Part model, mm, in its own coordinate system. A direction names the side the tool comes from. Give positions to 0.01 mm unless a question says otherwise; leave off trailing zeros. Order: outer loops, then holes, each group sorted by start corner. A loop starts at its lowest first (then second) coordinate and runs counter-clockwise, first axis right, second up. Notation, with made-up numbers: M 65,13 L 97,13 A12 cw 97,33 Z; hole C 1,-11.5 d6. An arc over 180 degrees is marked long. Return JSON: item names as keys, results as strings.
Autodesk Inventor part; units mm, degrees
ref_plane "YZ Plane" through (0, 0, 0) normal (1, 0, 0) x (0, 1, 0)
ref_plane "XZ Plane" through (0, 0, 0) normal (0, 1, 0) x (-1, 0, 0)
ref_plane "XY Plane" through (0, 0, 0) normal (0, 0, 1) x (1, 0, 0)
sketch "Sketch1" plane through (0, 0, 0) normal (0, 1, 0) x (-1, 0, 0)
  line L0 (0, 0) -> (68, 0)
  line L1 (68, 0) -> (68, -93)
  line L2 (68, -93) -> (0, -93)
  line L3 (0, -93) -> (0, 0)
  dimension "d0" = 93
  dimension "d1" = 68
extrude "Extrusion1" add sketch "Sketch1" along normal blind 8
fillet "Fillet1" radius 5 2 edges at (0, 4, -93) (-68, 4, -93)
fillet "Fillet2" radius 5 2 edges at (-68, 4, 0) (0, 4, 0)
sketch "Sketch2" plane through (0, 0, 0) normal (0, -1, 0) x (1, 0, 0)
  circle A0 centre (-7.8137, -81.5) radius 4
  circle A1 centre (-60.1863, -81.5) radius 4
  circle A2 centre (-60.1863, -11.5) radius 4
  circle A3 centre (-7.8137, -11.5) radius 4
  circle A4 centre (-34, -36) radius 4
  point P0 (0, 0)
  dimension "d27" = 70
  dimension "d28" = 52.3726
  dimension "d29" = 8
  dimension "d30" = 24.5
  dimension "d31" = 26.1863
  dimension "d32" = 11.5
  dimension "d33" = 7.8137
hole "Hole1" at (-7.8137, 0, -81.5) at (-60.1863, 0, -81.5) at (-60.1863, 0, -11.5) at (-7.8137, 0, -11.5) direction (0, 1, 0) diameter 5 end through all
sketch "Sketch3" plane through (0, 8, 0) normal (0, 1, 0) x (1, 0, 0)
  circle A0 centre (-34, 65) radius 11.8188 construction
  line L0 (-63, 0) -> (-5, 0)
  line L1 (0, 5) -> (0, 88)
  arc A1 (-27, 77.1244) -> (-34, 79) centre (-34, 65) ccw construction
  arc A2 (-26, 78.8564) -> (-34, 81) centre (-34, 65) ccw
  arc A3 (-28, 75.3923) -> (-34, 77) centre (-34, 65) ccw
  arc A4 (-28, 75.3923) -> (-26, 78.8564) centre (-27, 77.1244) ccw
  arc A5 (-34, 81) -> (-34, 77) centre (-34, 79) ccw
  line L2 (-27, 77.1244) -> (-34, 65) construction
  line L3 (-34, 65) -> (-34, 79) construction
  arc A6 (-41, 77.1244) -> (-46.1244, 72) centre (-34, 65) ccw construction
  arc A7 (-42, 78.8564) -> (-47.8564, 73) centre (-34, 65) ccw
  arc A8 (-40, 75.3923) -> (-44.3923, 71) centre (-34, 65) ccw
  arc A9 (-40, 75.3923) -> (-42, 78.8564) centre (-41, 77.1244) ccw
  arc A10 (-47.8564, 73) -> (-44.3923, 71) centre (-46.1244, 72) ccw
  arc A11 (-48, 65) -> (-46.1244, 58) centre (-34, 65) ccw construction
  arc A12 (-50, 65) -> (-47.8564, 57) centre (-34, 65) ccw
  arc A13 (-46, 65) -> (-44.3923, 59) centre (-34, 65) ccw
  arc A14 (-46, 65) -> (-50, 65) centre (-48, 65) ccw
  arc A15 (-47.8564, 57) -> (-44.3923, 59) centre (-46.1244, 58) ccw
  arc A16 (-41, 52.8756) -> (-34, 51) centre (-34, 65) ccw construction
  arc A17 (-42, 51.1436) -> (-34, 49) centre (-34, 65) ccw
  arc A18 (-40, 54.6077) -> (-34, 53) centre (-34, 65) ccw
  arc A19 (-40, 54.6077) -> (-42, 51.1436) centre (-41, 52.8756) ccw
  arc A20 (-34, 49) -> (-34, 53) centre (-34, 51) ccw
  line L4 (-5, 93) -> (-63, 93)
  arc A21 (-27, 52.8756) -> (-21.8756, 58) centre (-34, 65) ccw construction
  arc A22 (-26, 51.1436) -> (-20.1436, 57) centre (-34, 65) ccw
  arc A23 (-28, 54.6077) -> (-23.6077, 59) centre (-34, 65) ccw
  arc A24 (-28, 54.6077) -> (-26, 51.1436) centre (-27, 52.8756) ccw
  arc A25 (-20.1436, 57) -> (-23.6077, 59) centre (-21.8756, 58) ccw
  arc A26 (-20, 65) -> (-21.8756, 72) centre (-34, 65) ccw construction
  arc A27 (-18, 65) -> (-20.1436, 73) centre (-34, 65) ccw
  arc A28 (-22, 65) -> (-23.6077, 71) centre (-34, 65) ccw
  arc A29 (-22, 65) -> (-18, 65) centre (-20, 65) ccw
  arc A30 (-20.1436, 73) -> (-23.6077, 71) centre (-21.8756, 72) ccw
  point P0 (0, 0)
  dimension "d15" = 4
  dimension "d16" = 30
  dimension "d18" = 14
  dimension "d19" = 34
  dimension "d22" = 360
  dimension "d26" = 28
extrude "Extrusion2" cut sketch "Sketch3" against normal through all
properties part number "Z_platte_oben_new" material "PET Plastic"
Q1. Two-plate mould, pull along Z, no slides. Class faces 1 (the flat face through (-34, 4, 0)), 2 (the cylindrical face through (-6.29, 4.06, -79.52)), 3 (the flat face through (0, 4, -47)): +Z half, -Z half, draft (parallel to the pull), parting line (faces both ways), or undercut.
Established:
{"face 1": "+Z half", "face 2": "undercut", "face 3": "draft"}
Q2. Band-saw the part on A-A (z = -11.5). Give the cut face in (x, y).
Established:
{"outline": "M -68,0 L -62.69,0 L -62.69,8 L -68,8 Z; M -57.69,0 L -10.31,0 L -10.31,8 L -57.69,8 Z; M -5.31,0 L 0,0 L 0,8 L -5.31,8 Z"}
Q3. 3-axis set-ups, long thin cutter, end or side, ignore diameter. For faces 4 (the cylindrical face through (-66, 4, -92)), 5 (the cylindrical face through (-48, 4, -67)): which of +Z, -Z, +X, -X, +Y, -Y reach the whole face in a straight line?
Established:
{"face 4": "-Z, -X, +Y, -Y", "face 5": "+Y, -Y"}
Q4. Band-saw the part on B-B (x = -33). Give the cut face in (y, z).
Established:
{"outline": "M 0,-93 L 8,-93 L 8,-80.97 L 0,-80.97 Z; M 0,-76.96 L 8,-76.96 L 8,-52.73 L 0,-52.73 Z; M 0,-49.27 L 8,-49.27 L 8,0 L 0,0 Z"}
Q5. Probe line 1 along Z through (x, y) = (-60, 6); line 2 along X through (y, z) = (5.25, -11.5); line 3 along X through (y, z) = (5.75, -12.5). List the from-to ranges inside material, lowest first.
Established:
{"line 1": "z = -93 to -83.99, -79.01 to -13.99, -9.01 to 0", "line 2": "x = -68 to -62.69, -57.69 to -10.31, -5.31 to 0", "line 3": "x = -68 to -62.48, -57.9 to -10.1, -5.52 to 0"}
Q6. Band-saw the part on C-C (z = -68). Give the cut face in (x, y).
Established:
{"outline": "M -68,0 L -22.38,0 L -22.38,8 L -68,8 Z; M -18.28,0 L 0,0 L 0,8 L -18.28,8 Z"}
Q7. Band-saw the part on D-D (y = 5.5). Give the number of separate pieces and of enclosed holes in the cut face, then the cut area to 3 significant figures.
Established:
{"separate pieces": "1", "enclosed holes": "10", "area": "5,970 mm²"}
